Source: CAD feature listing. Evaluate the final solid. Frame: model axes, mm. A direction names the side the tool comes from. Round coordinates to 2 decimals unless told otherwise and drop trailing zeros. Order: outer loops, then holes, each group sorted by start corner. A loop starts at its lowest first (then second) coordinate and runs counter-clockwise, first axis right, second up. Notation, with made-up numbers: (41, -35) - (67, -35) arc R33 cw to (67, -5) - close; hole circle Ø7 at (37.25, 35). An arc over 180 degrees is marked (long way). Return JSON: item names as keys, results as strings. Group by question number.
1) Access query for faces 1 (the flat face through (231, 66.802, 13)), 2 (the flat face through (268.219, -137, 13)), 3 (the flat face through (288.544, -36, 13)). Directions: +Z, -Z, +X, -X, +Y, -Y. A direction counts if a zero-diameter tool reaches every point of the face in a straight line with its end or side. Return the directions, or none.
2) Contact query for flat-ended pins moving along their axis: P1, Ø10, axis at x = 27.5, z = 11, coming from the -Y side; P2, Ø3, axis at x = 244.5, z = 20.5, coming from the -Y side (3 decimals). Output: stop coordinate, or through.
3) Section A-A, the plane y = 36. Return loops of the section in (x, z).
4) Section B-B, the plane x = 13. Return loops of the section in (y, z), plus the area to 3 significant figures.
5) Mould query, pull axis Y, two halves, no side actions, for faces 4 (the flat face through (207.04, -137, 13)), 5 (the flat face through (182.372, -51, 13)), 6 (the flat face through (143, 73.152, 13)), 7 (the flat face through (13, -27.178, 13)). Classes: pulls with the +Y half, pulls with the -Y half, needs draft (parallel to the pull), parting line crosses it, or undercut.
6) Section C-C, the plane y = -119.5. Return loops of the section in (x, z).
7) Ray query, line 1 (Y direction, x = 117.5, z = 24.25); line 2 (Y direction, x = 276.5, z = 21.25) (3 decimals); line 3 (Y direction, x = 61, z = 4). Return the intervals inside material, ascending. Write a range as from..to.
8) Section D-D, the plane x = 116.5. Return loops of the section in (y, z), plus the area to 3 significant figures.
```python
from build123d import *

# Parameters (mm, degrees)
F0_W     = 2.54
F0_H     = 64.262
F0_W_2   = 58.928
F0_H_2   = 2.54
F0_W_3   = 9.906
F0_H_3   = 5.969
F0_W_4   = 5.969
F0_H_4   = 5.715
F0_H_5   = 49.022
F0_W_5   = 25.3746
F1_DEPTH = 25.4


# Not quite as in the source:
# - a feature names something its author has since deleted; it is built from what else it names


with BuildPart() as f1:
    # F0 (on Top) → F1 (new body)
    with BuildSketch(Plane.XY):
        Polygon((-6.35, 73.152), (-6.35, -82.55), (185.928, -82.55), (185.928, -143.0351776838), (207.0404606759, -143.0351776838), (207.0404606759, -131.445), (268.2187365532, -131.445), (268.2187365532, -142.524239029), (288.544, -142.524239029), (288.544, -81.915), (288.544, 73.152), align=None)
        Polygon((0, 61.5773126483), (0, 66.802), (77.6735246181, 66.802), (100.838, 66.802), (103.378, 66.802), (178.054, 66.802), (180.594, 66.802), (282.194, 66.802), (282.194, 48.7640425563), (282.194, 2.54), (282.194, 0), (282.194, -64.607180655), (282.194, -76.2), (282.194, -81.915), (282.194, -136.174239029), (274.5687365532, -136.174239029), (274.5687365532, -125.095), (200.6904606759, -125.095), (200.6904606759, -136.6851776838), (192.278, -136.6851776838), (192.278, -82.169), (192.278, -76.2), (182.372, -76.2), (176.022, -76.2), (153.67, -76.2), (151.13, -76.2), (77.216, -76.2), (74.676, -76.2), (52.324, -76.2), (49.784, -76.2), (0, -76.2), (0, -27.178), (0, -24.638), (0, 0), (0, 2.54), (0, 17.2067563981), (0, 18.169073388), (0, 22.6956792176), align=None, mode=Mode.SUBTRACT)
        Polygon((18.6906643212, 2.54), (0, 2.54), (0, 0), (78.0796, 0), (78.0796, 2.54), (68.6789600206, 2.54), (68.1948126652, 2.54), (29.4852126652, 2.54), (29.2154226812, 2.54), (29.2154226812, 1.9534120802), (20.0714226812, 1.9534120802), (20.0714226812, 2.54), (19.6596, 2.54), align=None)
        Polygon((103.378, 66.802), (100.838, 66.802), (100.838, 48.322211951), (100.838, 2.0835588062), (103.378, 2.0835588062), align=None)
        Polygon((180.594, 2.54), (178.054, 2.54), (126.6382832546, 2.54), (126.6382832546, 0), (200.914, 0), (200.914, 2.54), (198.7368017435, 2.54), align=None)
        with Locations((179.324, 34.671)):
            Rectangle(F0_W, F0_H)
        with Locations((252.73, 1.27)):
            Rectangle(F0_W_2, F0_H_2)
        Polygon((176.022, -72.2413137555), (176.022, -76.2), (182.372, -76.2), (182.372, -66.0237371922), (182.372, -29.6653471887), (182.372, -24.638), (176.022, -24.638), (176.022, -31.1945881695), (176.022, -37.9491113126), (176.022, -44.4958023727), (176.022, -51.689), (176.022, -58.7322562933), (176.022, -65.4867812991), align=None)
        with Locations((197.231, -79.1845)):
            Rectangle(F0_W_3, F0_H_3)
        with Locations((279.2095, -79.0575)):
            Rectangle(F0_W_4, F0_H_4)
        Polygon((151.13, -64.7879913449), (151.13, -76.2), (153.67, -76.2), (153.67, -72.2413137555), (153.67, -65.4867812991), (153.67, -58.7322562933), (153.67, -51.689), (153.67, -46.2308526039), (153.67, -44.4958023727), (153.67, -37.9491113126), (153.67, -31.1945881695), (153.67, -27.178), (151.13, -27.178), (151.13, -46.2308526039), align=None)
        Polygon((97.8137195742, -27.178), (151.13, -27.178), (153.67, -27.178), (153.67, -24.638), (97.8137195742, -24.638), align=None)
        with Locations((75.946, -51.689)):
            Rectangle(F0_W, F0_H_5)
        Polygon((71.8879923224, -27.178), (74.676, -27.178), (77.216, -27.178), (81.5490037203, -27.178), (81.5490037203, -24.638), (71.8879923224, -24.638), align=None)
        with Locations((51.054, -51.689)):
            Rectangle(F0_W, F0_H_5)
        Polygon((42.6438264549, -27.178), (49.784, -27.178), (52.324, -27.178), (55.1770441234, -27.178), (55.1770441234, -24.638), (42.6438264549, -24.638), align=None)
        with Locations((12.6873, -25.908)):
            Rectangle(F0_W_5, F0_H_2)
    extrude(amount=F1_DEPTH)


solid = f1.part
```
Geometry check:
{
 "1": {"face 1": "+Z, -Z", "face 2": "+Z, -Z, -Y", "face 3": "+Z, -Z, +X, +Y, -Y"},
 "2": {"P1": "y = -82.55", "P2": "y = -131.445"},
 "3": {"outline": "(-6.35, 0) - (0, 0) - (0, 25.4) - (-6.35, 25.4) - close; (100.84, 0) - (103.38, 0) - (103.38, 25.4) - (100.84, 25.4) - close; (178.05, 0) - (180.59, 0) - (180.59, 25.4) - (178.05, 25.4) - close; (282.19, 0) - (288.54, 0) - (288.54, 25.4) - (282.19, 25.4) - close"},
 "4": {"outline": "(-82.55, 0) - (-76.2, 0) - (-76.2, 25.4) - (-82.55, 25.4) - close; (-27.18, 0) - (-24.64, 0) - (-24.64, 25.4) - (-27.18, 25.4) - close; (0, 0) - (2.54, 0) - (2.54, 25.4) - (0, 25.4) - close; (66.8, 0) - (73.15, 0) - (73.15, 25.4) - (66.8, 25.4) - close", "area": "452 mm2"},
 "5": {"face 4": "needs draft", "face 5": "undercut", "face 6": "pulls with the +Y half", "face 7": "undercut"},
 "6": {"outline": "(185.93, 0) - (192.28, 0) - (192.28, 25.4) - (185.93, 25.4) - close; (282.19, 0) - (288.54, 0) - (288.54, 25.4) - (282.19, 25.4) - close"},
 "7": {"line 1": "-82.55..-76.2, -27.18..-24.64, 66.8..73.15", "line 2": "-142.524..-136.174, -81.915..-76.2, 0..2.54, 66.802..73.152", "line 3": "-82.55..-76.2, 0..2.54, 66.8..73.15"},
 "8": {"outline": "(-82.55, 0) - (-76.2, 0) - (-76.2, 25.4) - (-82.55, 25.4) - close; (-27.18, 0) - (-24.64, 0) - (-24.64, 25.4) - (-27.18, 25.4) - close; (66.8, 0) - (73.15, 0) - (73.15, 25.4) - (66.8, 25.4) - close", "area": "387 mm2"}
}
